Input: part model. Units: mm. Frame: model coordinates. Round coordinates to 2 decimals unless told otherwise and drop trailing zeros. Loops run counter-clockwise (first coordinate to the right, second up) from the corner with the lowest first, then second, coordinate; pieces in that order, holes last. Notation, with made-up numbers: M -2.5,-35.75 L 53.5,-35.75 A11 ccw 53.5,-27.75 Z; hole C -22.5,46 d5. An arc over 180 degrees is marked long. Use one line per item in the form item = value. Start each with the question number.
Q1. Ray query, line 1 along X through (y, z) = (-10, -0.85); line 2 along X through (y, z) = (-12.5, -0.45); line 3 along Y through (x, z) = (37.5, -0.3). Return the intervals inside material, ascending.
Q2. Section query A-A, the plane y = -10. Output: boundary loops of the cut face in (x, z).
Q3. Mould query, pull axis Y, two halves, no side actions, for faces 1 (the flat face through (25, -26, -2)), 2 (the cylindrical face through (8.52, -12.32, -0.99)), 3 (the flat face through (25, 0, -1)). Classes: pulls with the +Y half, pulls with the -Y half, needs draft (parallel to the pull), parting line crosses it, or undercut.
Q4. Section query C-C, the plane z = -1.3. Output: boundary loops of the cut face in (x, y).
Q5. Section query D-D, the plane y = -56. Output: boundary loops of the cut face in (x, z), and give its area (3 significant figures).
Q6. First-contact query: P1, Ø3.5, axis at x = 12.99, y = -40.95, coming from the -Z side. Flat tip, straight axial feed; report the tip coordinate or a pass-through.
Q7. Section query B-B, the plane x = 40. Output: boundary loops of the cut face in (y, z), and give its area (3 significant figures).
```python
from build123d import *

# Parameters (mm, degrees)
EXTRUDE_1_DEPTH   = 2
HOLE_WIZARD_M51_D = 5.5
CHAMFER_1_SIZE    = 2.5


with BuildPart() as part:
    # Эскиз3 → Бобышка-Вытянуть1 (new body)
    with BuildSketch(Plane(origin=(0, 0, 0), x_dir=(1, 0, 0), z_dir=(0, 0, -1))):
        Polygon((0, 0), (50, 0), (50, 50.773502692), (40, 68.094010768), (0, 45), align=None)
    extrude(amount=EXTRUDE_1_DEPTH)

    # Отверстие с зазором M51 (through all)
    with Locations(Plane(origin=(0, 0, -2), x_dir=(1, 0, 0), z_dir=(0, 0, -1))):
        with Locations((10, 10), (40, 10), (12.990381057, 40.952994616), (36.339745962, 54.43375673)):
            Hole(HOLE_WIZARD_M51_D / 2)

    # Фаска1
    chamfer_1_edges = [part.edges().sort_by_distance(p)[0] for p in [
        (40, -68.094010768, -1),
        (50, 0, -1),
        (0, 0, -1),
    ]]
    chamfer(chamfer_1_edges, length=CHAMFER_1_SIZE)


solid = part.part
```
Results found:
q1.line_1 = 0 to 7.25, 12.75 to 37.25, 42.75 to 50
q1.line_2 = 0 to 8.85, 11.15 to 38.85, 41.15 to 50
q1.line_3 = -66.65 to -56.93, -51.94 to -11.15, -8.85 to 0
q2.outline = M 0,-2 L 7.25,-2 L 7.25,0 L 0,0 Z; M 12.75,-2 L 37.25,-2 L 37.25,0 L 12.75,0 Z; M 42.75,-2 L 50,-2 L 50,0 L 42.75,0 Z
q3.face_1 = needs draft
q3.face_2 = undercut
q3.face_3 = pulls with the +Y half
q4.outline = M 0,-45 L 37.83,-66.84 L 41.25,-65.93 L 50,-50.77 L 50,-2.5 L 47.5,0 L 2.5,0 L 0,-2.5 Z; hole C 10,-10 d5.5; hole C 12.99,-40.95 d5.5; hole C 36.34,-54.43 d5.5; hole C 40,-10 d5.5
q5.outline = M 19.05,-2 L 34.08,-2 L 34.08,0 L 19.05,0 Z; M 38.6,-2 L 46.98,-2 L 46.98,0 L 38.6,0 Z
q5.area = 46.8 mm²
q6.P1 = through
q7.outline = M -66.26,-2 L -12.75,-2 L -12.75,0 L -66.26,0 Z; M -7.25,-2 L 0,-2 L 0,0 L -7.25,0 Z
q7.area = 122 mm²
